Verification items for the finished model (mm, model axes). A direction names the side the tool comes from. Give positions to 0.01 mm unless a question says otherwise; leave off trailing zeros. Loops run counter-clockwise (first coordinate to the right, second up) from the corner with the lowest first, then second, coordinate; pieces in that order, holes last. Notation, with made-up numbers: (-24.75, 21.25) - (26.25, 21.25) arc R37 cw to (26.25, 60.25) - close; hole circle Ø1 at (50, 72). An arc over 180 degrees is marked (long way). Use one line per item in the form item = value.
```python
from build123d import *

# Parameters (mm, degrees)
SKETCH1_R           = 2.5
BOSS_EXTRUDE1_DEPTH = 3
BOSS_EXTRUDE2_DEPTH = 5
FILLET1_R           = 1.8


with BuildPart() as part:
    # Sketch1 → Boss-Extrude1 (new, symmetric)
    with BuildSketch(Plane(origin=(0, 0, 0), x_dir=(0, 1, 0), z_dir=(0, 0, 1))):
        with BuildLine():
            ThreePointArc((-10.825318, 6.25), (0, -12.5), (10.825318, 6.25))
            ThreePointArc((10.825318, 6.25), (9.150635, 12.5), (10.825318, 18.75))
            ThreePointArc((10.825318, 18.75), (0, 37.5), (-10.825318, 18.75))
            ThreePointArc((-10.825318, 18.75), (-9.150635, 12.5), (-10.825318, 6.25))
        make_face()
        with Locations(Location((0, 0, 0), (0, 0, 270))):
            Circle(SKETCH1_R, mode=Mode.SUBTRACT)
        with Locations(Location((-7.5, 25, 0), (0, 0, 270))):
            Circle(SKETCH1_R, mode=Mode.SUBTRACT)
    extrude(amount=BOSS_EXTRUDE1_DEPTH, both=True)

    # Sketch2 → Boss-Extrude2 (add, symmetric)
    with BuildSketch(Plane(origin=(0, 0, 0), x_dir=(0, 1, 0), z_dir=(0, 0, 1))):
        with BuildLine():
            ThreePointArc((0, 35.307764), (0.727582, 36.850798), (2.380952, 37.271148))
            ThreePointArc((2.380952, 37.271148), (3.841576, 36.895053), (5.24627, 36.345777))
            Line((5.24627, 36.345777), (36.995968, 21.664764))
            ThreePointArc((36.995968, 21.664764), (42.261052, 20.064281), (47.763018, 19.959286))
            Line((47.763018, 19.959286), (127.25476, 29.458153))
            ThreePointArc((127.25476, 29.458153), (128.486622, 30.086985), (129.015888, 31.364792))
            ThreePointArc((129.015888, 31.364792), (141.598901, 36.577029), (137.399882, 23.620645))
            Line((137.399882, 23.620645), (51.992546, 13.414894))
            ThreePointArc((51.992546, 13.414894), (44.103222, 13.1), (36.262693, 14.030963))
            Line((36.262693, 14.030963), (11.019597, 19.075031))
            Line((11.019597, 19.075031), (2.780641, 23.156138))
            ThreePointArc((2.780641, 23.156138), (0.751659, 25), (0, 27.636589))
            Line((0, 27.636589), (0, 35.307764))
        make_face()
    extrude(amount=BOSS_EXTRUDE2_DEPTH, both=True)

    # Fillet1
    fillet1_edges = [part.edges().sort_by_distance(p)[0] for p in [
        (-36.850798, 0.727582, 5),
        (-21.115584, 6.900119, -5),
        (-31.472177, 0, -5),
        (-25, 0.751659, -5),
        (-16.552997, 23.641145, 5),
        (-13.1, 44.103222, -5),
        (-18.51777, 94.696214, -5),
        (-36.577029, 141.598901, -5),
        (-30.086985, 128.486622, 5),
        (-24.70872, 87.508889, 5),
        (-20.064281, 42.261052, 5),
        (-29.00527, 21.121119, 5),
        (-36.895053, 3.841576, -5),
        (-31.472177, 0, 5),
        (-25, 0.751659, 5),
        (-21.115584, 6.900119, 5),
        (-13.1, 44.103222, 5),
        (-18.51777, 94.696214, 5),
        (-36.577029, 141.598901, 5),
        (-36.895053, 3.841576, 5),
        (-36.850798, 0.727582, -5),
        (-29.00527, 21.121119, -5),
        (-20.064281, 42.261052, -5),
        (-24.70872, 87.508889, -5),
        (-30.086985, 128.486622, -5),
        (-16.552997, 23.641145, -5),
    ]]
    fillet(fillet1_edges, radius=FILLET1_R)


solid = part.part
```
1. Depth check by flat-ended pin: pin 1 Ø3 at (x, y) = (-25, -7.5) entering from -Z; pin 2 Ø1 at (x, z) = (-13.5, -3) entering from -Y; pin 3 Ø20 at (x, y) = (-6, -3) entering from +Z; pin 4 Ø6 at (y, z) = (18, -4) entering from -X. Enter the tip coordinate at first touch or a pass-through.
Result set:
pin_1 = through
pin_2 = -9.24
pin_3 = 3
pin_4 = -31.8
2. Section check B-B, the plane z = 0. State how many separate pieces and enclosed holes the cut face has, then the cut area to 3 significant figures.
Result set:
separate_pieces = 1
enclosed_holes = 2
area = 2,120 mm²
3. Draft check along X on faces 6 (the cylindrical face through (-17.12, 23.57, 4.49)), 7 (the cylindrical face through (-0.54, -2.44, -0.04)), 8 (the flat face through (-19, 67, 5)). Enter one of: released by +X, released by -X, zero draft, split by the parting line, or undercut.
Result set:
face_6 = released by +X
face_7 = undercut
face_8 = zero draft
4. Section check A-A, the plane x = 0. Record the cut outline in (y, z), then the cut area to 3 significant figures.
Result set:
outline = (-12.5, -3) - (-2.5, -3) - (-2.5, 3) - (-12.5, 3) - close; (2.5, -3) - (12.5, -3) - (12.5, 3) - (2.5, 3) - close
area = 120 mm²
5. Scan lines: probe 1 along Y at (x, z) = (0, 0.2); probe 2 along Z at (x, y) = (-25, -1); probe 3 along X at (y, z) = (44.5, 3.75). Record each from-to range of solid material in increasing order.
Result set:
probe_1 = -12.5 to -2.5, 2.5 to 12.5
probe_2 = -3 to 3
probe_3 = -19.75 to -13.17
6. Tool access check on faces 1 (the cylindrical face through (-28.411, 21.116, 4.487)), 2 (the flat face through (-29.108, 20.899, 0.045)), 3 (the cylindrical face through (-13.096, 44.214, 0.045)), 4 (the cylindrical face through (-28.411, 21.116, -4.487)), 5 (the flat face through (-19, 67, -5)). Record the directions out of +Z, -Z, +X, -X, +Y, -Y that give a thin tool (end or side, any length) a straight path to the whole face; none if there is none.
Result set:
face_1 = +Z, -X
face_2 = +Z, -Z, -X
face_3 = +Z, -Z, +X
face_4 = -Z, -X
face_5 = -Z, +X, -X, +Y, -Y
7. Section check C-C, the plane y = -7.5. Record the cut outline in (x, z), then the cut area to 3 significant figures.
Result set:
outline = (-35, -3) - (-27.5, -3) - (-27.5, 3) - (-35, 3) - close; (-22.5, -3) - (10, -3) - (10, 3) - (-22.5, 3) - close
area = 240 mm²
